from build123d import *

# Parameters (mm, degrees)
SKETCH1_R           = 127
SKETCH1_R_2         = 63.5
BOSS_EXTRUDE1_DEPTH = 5.334
SKETCH2_W           = 50.8
SKETCH2_H           = 50.8
WHEELSCUT_DEPTH     = 180.684310823
SKETCH3_W           = 4.826
SKETCH3_H           = 6.35
TOPBOTTOMCUT_DEPTH  = 178.879992006
SKETCH4_W           = 6.35
SKETCH4_H           = 4.826
SIDECUT_DEPTH       = 178.879992006
SKETCH14_R          = 3.175
BOLTHOLES_DEPTH     = 178.879992006
SKETCH15_W          = 2.4638
SKETCH15_H          = 19.05
SKETCH15_W_2        = 5.334
MOTORMOUNTS_DEPTH   = 178.879992006


with BuildPart() as part:
    # Sketch1 → Boss-Extrude1 (new body)
    # profile 1 of 3: a face of its own
    with BuildSketch(Plane.XY):
        Circle(SKETCH1_R)
        Circle(SKETCH1_R_2, mode=Mode.SUBTRACT)
    # profile 2 of 3: a face of its own
    with BuildSketch(Plane.XY):
        with BuildLine():
            Line((-40.299999918, -49.073006904), (-40.299999918, 49.073006904))
            ThreePointArc((-40.299999918, 49.073006904), (-63.5, 0), (-40.299999918, -49.073006904))
        make_face()
    # profile 3 of 3: a face of its own
    with BuildSketch(Plane.XY):
        with BuildLine():
            ThreePointArc((63.5, 0), (57.407752067, 27.140375874), (40.299999918, 49.073006904))
            Line((40.299999918, 49.073006904), (40.299999918, -49.073006904))
            ThreePointArc((40.299999918, -49.073006904), (57.407752067, -27.140375874), (63.5, 0))
        make_face()
    extrude(amount=BOSS_EXTRUDE1_DEPTH)

    # Sketch2 → WheelsCut (cut, through all)
    with BuildSketch(Plane.XY.offset(5.334)):
        with Locations((-127, 0)):
            Rectangle(SKETCH2_W, SKETCH2_H)
        with Locations((127, 0)):
            Rectangle(SKETCH2_W, SKETCH2_H)
    extrude(amount=-WHEELSCUT_DEPTH, mode=Mode.SUBTRACT)

    # Sketch3 → TopBottomCut (cut, through all)
    with BuildSketch(Plane.XY.offset(5.334)):
        with Locations((-17.653, 89.789)):
            Rectangle(SKETCH3_W, SKETCH3_H)
        with Locations((17.653, 89.789)):
            Rectangle(SKETCH3_W, SKETCH3_H)
        with Locations((0, -89.789)):
            Rectangle(SKETCH3_W, SKETCH3_H)
        with Locations((0, 89.789)):
            Rectangle(SKETCH3_W, SKETCH3_H)
        with Locations((17.653, -89.789)):
            Rectangle(SKETCH3_W, SKETCH3_H)
        with Locations((-17.653, -89.789)):
            Rectangle(SKETCH3_W, SKETCH3_H)
    extrude(amount=-TOPBOTTOMCUT_DEPTH, mode=Mode.SUBTRACT)

    # Sketch4 → SideCut (cut, through all)
    with BuildSketch(Plane.XY.offset(5.334)):
        with Locations((-80.645, 47.625)):
            Rectangle(SKETCH4_W, SKETCH4_H)
        with Locations((-80.645, 34.925)):
            Rectangle(SKETCH4_W, SKETCH4_H)
        with Locations((-80.645, 60.325)):
            Rectangle(SKETCH4_W, SKETCH4_H)
        with Locations((80.645, 60.325)):
            Rectangle(SKETCH4_W, SKETCH4_H)
        with Locations((80.645, 47.625)):
            Rectangle(SKETCH4_W, SKETCH4_H)
        with Locations((80.645, 34.925)):
            Rectangle(SKETCH4_W, SKETCH4_H)
    extrude(amount=-SIDECUT_DEPTH, mode=Mode.SUBTRACT)

    # Sketch14 → BoltHoles (cut, through all)
    with BuildSketch(Plane.XY.offset(5.334)):
        with Locations((-76.2, -78.74)):
            Circle(SKETCH14_R)
        with Locations((-50.8, 78.74)):
            Circle(SKETCH14_R)
        with Locations(Location((76.2, -78.74, 0), (0, 0, 180))):
            Circle(SKETCH14_R)
        with Locations(Location((50.8, 78.74, 0), (0, 0, 180))):
            Circle(SKETCH14_R)
    extrude(amount=-BOLTHOLES_DEPTH, mode=Mode.SUBTRACT)

    # Sketch15 → MotorMounts (cut, through all)
    with BuildSketch(Plane.XY.offset(5.334)):
        with Locations((-100.3681, -41.275)):
            Rectangle(SKETCH15_W, SKETCH15_H)
        with Locations((-100.3681, 0)):
            Rectangle(SKETCH15_W, SKETCH15_H)
        with Locations((-78.469199932, 0)):
            Rectangle(SKETCH15_W_2, SKETCH15_H)
        with Locations((-42.966999918, 0)):
            Rectangle(SKETCH15_W_2, SKETCH15_H)
        with Locations((-78.469199932, -41.275)):
            Rectangle(SKETCH15_W_2, SKETCH15_H)
        with Locations((-42.966999918, -41.275)):
            Rectangle(SKETCH15_W_2, SKETCH15_H)
        with Locations((42.966999918, -41.275)):
            Rectangle(SKETCH15_W_2, SKETCH15_H)
        with Locations((78.469199932, -41.275)):
            Rectangle(SKETCH15_W_2, SKETCH15_H)
        with Locations((100.3681, -41.275)):
            Rectangle(SKETCH15_W, SKETCH15_H)
        with Locations((42.966999918, 0)):
            Rectangle(SKETCH15_W_2, SKETCH15_H)
        with Locations((78.469199932, 0)):
            Rectangle(SKETCH15_W_2, SKETCH15_H)
        with Locations((100.3681, 0)):
            Rectangle(SKETCH15_W, SKETCH15_H)
    extrude(amount=-MOTORMOUNTS_DEPTH, mode=Mode.SUBTRACT)


solid = part.part
Verification items for the finished model (mm, model axes). A direction names the side the tool comes from. Give positions to 0.01 mm unless a question says otherwise; leave off trailing zeros. Write each loop counter-clockwise with the first axis right and the second up, starting at its lowest first coordinate (ties: lowest second). Pieces come first, ordered by that corner, then holes. Notation, with made-up numbers: (-34.5, 45) - (-10.5, 45) arc R20 cw to (-10.5, 70) - close; hole circle Ø4 at (-7.75, -40). An arc over 180 degrees is marked (long way). Answer as CSV lines item,"result". Start each with the question number.
1. Thickness scan on line 1 (X direction, y = 6.5, z = 1.05); line 2 (Y direction, x = 76.2, z = 3.6) (3 decimals); line 3 (X direction, y = -14, z = 1.4). Record the ranges inside material, lowest first.
2. Sectioned sample at D-D (z = 3.45). Count the separate pieces of the cut face and the enclosed holes in it, then the cut area to 3 significant figures.
3. Draft check along Y on faces 1 (the face through (-0.611, -63.497, 2.63)), 2 (the face through (-2.435, -126.977, 2.63)), 3 (the face through (-57, 2, 0)), 4 (the face through (74.493, -81.417, 2.704)). Enter one of: pulls with the +Y half, pulls with the -Y half, needs draft (parallel to the pull), parting line crosses it, or undercut.
4. Depth check by flat-ended pin: pin 1 (2.5 mm diameter, centred on x = -79, z = 4, fed in from -Y); pin 2 (2.5 mm diameter, centred on y = 59.5, z = 3.5, fed in from +X); pin 3 (1.6 mm diameter, centred on y = 1, z = 1.5, fed in from +X). Enter the tip coordinate at first touch or a pass-through.
5. Sectioned sample at B-B (x = 23.5). Record the boundary of the cut face in (y, z).
6. Sectioned sample at C-C (y = -78.74). Record the boundary of the cut face in (x, z) (3 decimals), then the cut area to 3 significant figures.
7. Set-up check for faces 5 (the face through (2.435, 126.977, 2.63)), 6 (the face through (0.611, 63.497, 2.63)): record each of +Z, -Z, +X, -X, +Y, -Y from which the full face is reachable in a straight line by a thin tool's end or side.
8. Sectioned sample at A-A (y = -20). Record the boundary of the cut face in (x, z), then the cut area to 3 significant figures.
Derived:
1,line 1,"-99.14 to -81.14, -75.8 to -45.63, 45.63 to 75.8, 81.14 to 99.14"
1,line 2,"-101.6 to -81.915, -75.565 to -50.8, -31.75 to -9.525, 9.525 to 101.6"
1,line 3,"-101.6 to -40.3, 40.3 to 101.6"
2,separate pieces,"1"
2,enclosed holes,"23"
2,area,"37,200 mm²"
3,face 1,"undercut"
3,face 2,"pulls with the -Y half"
3,face 3,"needs draft"
3,face 4,"undercut"
4,pin 1,"y = -100.42"
4,pin 2,"x = 112.85"
4,pin 3,"x = 99.14"
5,outline,"(-124.81, 0) - (-58.99, 0) - (-58.99, 5.33) - (-124.81, 5.33) - close; (58.99, 0) - (124.81, 0) - (124.81, 5.33) - (58.99, 5.33) - close"
6,outline,"(-99.644, 0) - (-79.375, 0) - (-79.375, 5.334) - (-99.644, 5.334) - close; (-73.025, 0) - (73.025, 0) - (73.025, 5.334) - (-73.025, 5.334) - close; (79.375, 0) - (99.644, 0) - (99.644, 5.334) - (79.375, 5.334) - close"
6,area,"995 mm²"
7,face 5,"+Z, -Z, +Y"
7,face 6,"+Z, -Z"
8,outline,"(-101.6, 0) - (-40.3, 0) - (-40.3, 5.33) - (-101.6, 5.33) - close; (40.3, 0) - (101.6, 0) - (101.6, 5.33) - (40.3, 5.33) - close"
8,area,"654 mm²"
